Source: CAD feature listing. Evaluate the final solid. Frame: model axes, mm. A direction names the side the tool comes from. Give positions to 0.01 mm unless a question says otherwise; leave off trailing zeros. Loops run counter-clockwise (first coordinate to the right, second up) from the corner with the lowest first, then second, coordinate; pieces in that order, holes last. Notation, with made-up numbers: (22, -21) -> (58, -21) arc R31 cw to (58, 14) -> close; hole circle Ø1 at (17.25, 54). An arc over 180 degrees is marked (long way). Return JSON: item names as keys, results as strings. Group by question number.
(1) Ray query, line 1 (X direction, y = 121, z = 13.7); line 2 (Z direction, x = -15, y = 37.6); line 3 (Z direction, x = -10.75, y = 147). Return the intervals inside material, ascending. Write a range as from..to.
(2) Cut plane B-B on x = -17.75. Return loops of the section in (y, z).
(3) Cut plane A-A on y = 151. Return loops of the section in (x, z), then the cut area to 3 significant figures.
(4) Cut plane D-D on y = 121. Return loops of the section in (x, z).
(5) Pin query (flat end, axial travel): pin 1 (2.5 mm diameter, centred on x = -15, y = 151, fed in from -Z); pin 2 (1 mm diameter, centred on x = -17.5, y = 138.5, fed in from -Z); pin 3 (0.9 mm diameter, centred on x = -15.5, y = 121.5, fed in from +Z); pin 4 (10 mm diameter, centred on y = 100.5, z = 3.5, fed in from +X). Return the tip coordinate at first contact, or that it passes through.
(6) Cut plane C-C on z = -9.5. Return loops of the section in (x, y), then the cut area to 3 significant figures.
(7) Access query for faces 5 (the face through (-10, 82, 0)), 6 (the face through (-15, 121, 5)), 7 (the face through (-14.93, 59.393, -10.895)), 8 (the face through (-16.5, 35.96, 7.07)), 9 (the face through (-15, 143, 5)). Directions: +Z, -Z, +X, -X, +Y, -Y. A direction counts if a zero-diameter tool reaches every point of the face in a straight line with its end or side. Return the directions, or none.
(8) Draft query along Y for faces 1 (the face through (-14.93, 84.17, -9.79)), 2 (the face through (-14.93, 107.95, 3.54)), 3 (the face through (-15, 96, 15)), 4 (the face through (-15.195, 122.487, 6.135)). Return one class per face: released by +Y, released by -Y, zero draft, split by the parting line, or undercut.
Autodesk Inventor part; units mm, degrees
ref_plane "작업 평면1" through (-15, 23, -25) normal (-1, 0, 0) x (0, 0, 1)
ref_plane "YZ Plane" through (0, 0, 0) normal (1, 0, 0) x (0, 1, 0)
ref_plane "XZ Plane" through (0, 0, 0) normal (0, 1, 0) x (-1, 0, 0)
sketch "스케치1" plane through (0, 0, 0) normal (0, 0, 1) x (1, 0, 0)
  line L0 (-5, -33) -> (5, -33)
  line L1 (5, -33) -> (5, 33)
  line L2 (5, 33) -> (-5, 33)
  line L3 (-5, 33) -> (-5, -33)
  line L4 (-5, -33) -> (5, 33) construction
  line L5 (5, -33) -> (-5, 33) construction
  line L6 (-5, 33) -> (-35, 33)
  line L7 (-35, 33) -> (-35, 23)
  line L8 (-35, 23) -> (-5, 23)
  line L9 (-5, 23) -> (-5, 33)
  line L10 (0, 0) -> (-11.0402, 0)
  line L11 (-5, -33) -> (-35, -33)
  line L12 (-35, -33) -> (-35, -23)
  line L13 (-35, -23) -> (-5, -23)
  point P0 (-5, 23)
  point P1 (-5, -23)
  dimension "d0" = 66
  dimension "d1" = 10
  dimension "d2" = 10
  dimension "d3" = 30
extrude "돌출1" add sketch "스케치1" along normal mid plane 50
sketch "스케치2" plane through (0, 0, 25) normal (0, 0, 1) x (1, 0, 0)
  circle A0 centre (-15, 183) radius 14
  line L0 (-35, 33) -> (-35, 23)
  line L1 (-35, 33) -> (-28.9889, 183.5585)
  line L2 (5, 33) -> (-35, 33)
  line L3 (-15, 33) -> (-15, 183) construction
  line L4 (5, 33) -> (-1.0111, 183.5585)
  point P0 (0, 0)
  dimension "d6" = 28
  dimension "d7" = 150
extrude "돌출2" add sketch "스케치2" against normal blind 10
ref_plane "작업 평면1" through (-15, 23, -25) normal (-1, 0, 0) x (0, 0, 1)
sketch "스케치3" plane through (-15, 23, -25) normal (-1, 0, 0) x (0, 0, 1)
  line L0 (40, 160.5585) -> (40, 10)
  line L1 (0, 10) -> (40, 10)
  line L2 (40, 144.5585) -> (0, 10)
  line L3 (45.7513, 142.8488) -> (8.0431, 16)
  line L4 (8.0431, 16) -> (34, 16)
  line L5 (34, 16) -> (34, 160.5585)
  line L6 (34, 16) -> (20, 56.2226)
  line L7 (34, 34.2526) -> (22.9265, 66.0672)
  point P0 (25, -23)
  point P1 (34, 103.318)
  point P2 (34, 124.3747)
  point P3 (40, 123.5018)
  dimension "d10" = 16
  dimension "d11" = 6
  dimension "d12" = 6
extrude "돌출3" add sketch "스케치3" along normal mid plane 10 contours L0 L3 L5 L2 | L0 L1 L2 L5 L3 | L7 L5 L6 L3
sketch "스케치4" plane through (0, 0, 25) normal (0, 0, 1) x (1, 0, 0)
  line L0 (-35, 33) -> (-28.9889, 183.5585)
  line L1 (5, 33) -> (-1.0111, 183.5585)
  line L2 (-35, 33) -> (5, 33)
  arc A0 (-1.0111, 183.5585) -> (-28.9889, 183.5585) centre (-15, 183) ccw
  line L3 (-7.0064, 183.3192) -> (-1.2443, 39)
  line L4 (-1.2443, 39) -> (-28.7557, 39)
  line L5 (-28.7557, 39) -> (-22.9936, 183.3192)
  arc A1 (-7.0064, 183.3192) -> (-22.9936, 183.3192) centre (-15, 183) ccw
  line L6 (-1.2443, 39) -> (-27.6994, 65.4551)
  line L7 (-1.5972, 47.8382) -> (-27.3737, 73.6146)
  line L8 (-27.3737, 73.6146) -> (-3.5765, 97.4118)
  line L9 (-3.9022, 105.5713) -> (-27.0208, 82.4528)
  line L10 (-3.9022, 105.5713) -> (-25.2456, 126.9147)
  line L11 (-25.2456, 126.9147) -> (-5.5411, 146.6192)
  line L12 (-5.5411, 146.6192) -> (-23.7326, 164.8107)
  line L13 (-23.7326, 164.8107) -> (-6.2674, 164.8107)
  line L14 (-21.003, 131.1573) -> (-4.2551, 114.4095)
  line L15 (-15.2473, 164.8107) -> (-5.894, 155.4574)
  line L16 (-24.8927, 135.7528) -> (-9.7837, 150.8618)
  point P0 (0, 0)
  point P1 (-5.2153, 138.4597)
  dimension "d15" = 6
  dimension "d16" = 45
  dimension "d17" = 6
  dimension "d18" = 90
  dimension "d19" = 6
  dimension "d23" = 6
extrude "돌출4" cut sketch "스케치4" against normal blind 10 contours L3 L15 L13 | L12 L16 L5 | L3 L14 L11 | L10 L9 L5 | L3 L7 L8 | L6 L4 L5
sketch "스케치5" plane through (5, -33, -25) normal (1, 0, 0) x (0, 0, -1)
  line L0 (-118.3974, 269.5393) -> (141.4613, 269.5393)
  line L1 (141.4613, 269.5393) -> (141.4613, -32.7297)
  line L2 (141.4613, -32.7297) -> (-118.3974, -32.7297)
  line L3 (-118.3974, -32.7297) -> (-118.3974, 269.5393)
  line L4 (-40, 216.5585) -> (-40, 66)
  line L5 (-40, 66) -> (56.641, 66)
  line L6 (56.641, 66) -> (56.641, 208.6229)
  line L7 (56.641, 208.6229) -> (-40, 208.6229)
  line L8 (-40, 208.6229) -> (-40, 66)
  point P0 (-25, 33)
extrude "돌출5" cut sketch "스케치5" against normal blind 128.75
sketch "스케치6" plane through (-20, 33, -25) normal (0, -1, 0) x (1, 0, 0)
  circle A0 centre (5, 8) radius 1.5
  line L0 (0, 0) -> (10, 0)
  line L1 (10, 0) -> (10, 40)
  circle A1 centre (5, 20) radius 1.5
  circle A2 centre (5, 32) radius 1.5
  point P0 (20, 25)
  point P1 (5, 0)
  dimension "d27" = 3
  dimension "d28" = 8
  dimension "d31" = 12
extrude "돌출6" cut sketch "스케치6" against normal up to surface (6 mm away)
sketch "스케치7" plane through (-10, 23, -25) normal (1, 0, 0) x (0, 0, -1)
  line L0 (-40, 144.5585) -> (-30, 144.5585)
  line L1 (-30, 144.5585) -> (-30, 110.9189)
  line L2 (-40, 144.5585) -> (0, 10)
  point P0 (-25, -23)
  point P1 (-39.8767, 144.1437)
  dimension "d38" = 10
extrude "돌출7" add sketch "스케치7" against normal blind 10
sketch "스케치8" plane through (0, 0, 15) normal (0, 0, 1) x (1, 0, 0)
  circle A0 centre (-15, 90) radius 1.5
  circle A1 centre (-15, 121) radius 1.5
  circle A2 centre (-15, 151) radius 1.5
  line L0 (-10, 33) -> (-20, 33)
  line L1 (-10, 167.5585) -> (-20, 167.5585)
  point P0 (0, 0)
  point P1 (-15, 167.5585)
  dimension "d43" = 3
  dimension "d44" = 3
  dimension "d45" = 3
  dimension "d46" = 30
  dimension "d47" = 31
  dimension "d48" = 57
extrude "돌출8" cut sketch "스케치8" against normal blind 10
sketch "스케치9" plane through (-10, 167.5585, 15) normal (0, 1, 0) x (1, 0, 0)
  line L0 (0, 10) -> (0, 0)
  line L1 (0, 10) -> (-10, 10)
  line L2 (-10, 0) -> (-10, 10)
  line L3 (0, 0) -> (-10, 0)
  point P0 (10, 15)
extrude "돌출9" cut sketch "스케치9" against normal blind 10
fillet "모깎기3" radius 5 1 edges at (-15, 157.5585, 5)
properties part number "전체 형상"
Answers:
{
 "1": {"line 1": "-20..-16.5, -13.5..-10", "line 2": "-23.63..-18.5, -15.5..-6.5, -3.5..5.5, 8.5..15", "line 3": "5..15"},
 "2": {"outline": "(33, -25) -> (133.92, 5) -> (152.56, 5) arc R5 ccw to (157.56, 10) -> (157.56, 15) -> (33, 15) -> close; hole (39, -16.96) -> (79.22, -5) -> (39, 9) -> close; hole (57.25, 9) -> (89.07, -2.07) -> (126.32, 9) -> close"},
 "3": {"outline": "(-20, 5) -> (-16.5, 5) -> (-16.5, 15) -> (-20, 15) -> close; (-13.5, 5) -> (-10, 5) -> (-10, 15) -> (-13.5, 15) -> close", "area": "70.0 mm²"},
 "4": {"outline": "(-20, 1.16) -> (-10, 1.16) -> (-10, 7.42) -> (-13.5, 7.42) -> (-13.5, 5) -> (-16.5, 5) -> (-16.5, 7.42) -> (-20, 7.42) -> close; (-20, 9) -> (-16.5, 9) -> (-16.5, 15) -> (-20, 15) -> close; (-13.5, 9) -> (-10, 9) -> (-10, 15) -> (-13.5, 15) -> close"},
 "5": {"pin 1": "through", "pin 2": "z = 5", "pin 3": "z = 5", "pin 4": "x = -10"},
 "6": {"outline": "(-20, 33) -> (-10, 33) -> (-10, 39) -> (-20, 39) -> close; (-20, 64.08) -> (-10, 64.08) -> (-10, 85.14) -> (-20, 85.14) -> close", "area": "271 mm²"},
 "7": {"face 5": "+Z, -Z, +X, +Y, -Y", "face 6": "+Z", "face 7": "+X, -X", "face 8": "-Y", "face 9": "-Z, +X, -X, +Y"},
 "8": {"face 1": "released by +Y", "face 2": "undercut", "face 3": "zero draft", "face 4": "undercut"}
}
